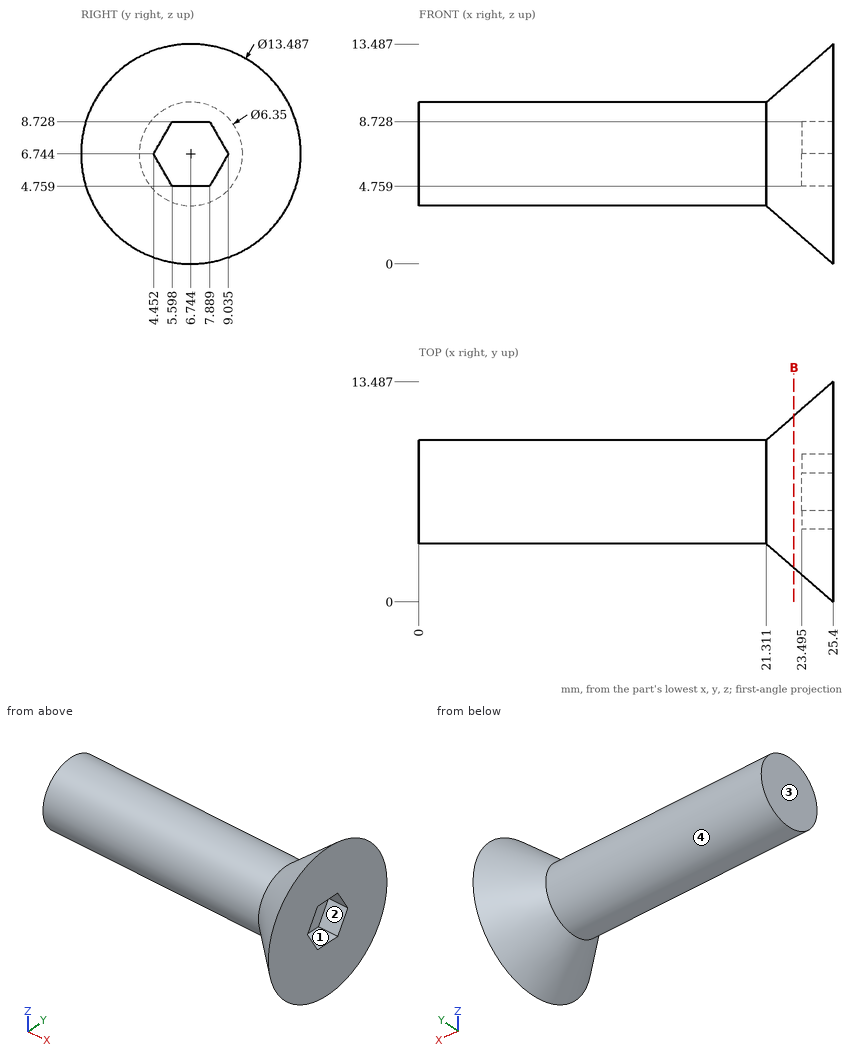
Source: three-view drawing plus pictorial views. Frame: mm from the lowest corner of the part. Give positions to 0.01 mm unless a question says otherwise; leave off trailing zeros. Order: outer loops, then holes, each group sorted by start corner. A loop starts at its lowest first (then second) coordinate and runs counter-clockwise, first axis right, second up. Notation, with made-up numbers: (-37.75, 26.25) - (-13.75, 26.25) arc R26 cw to (-13.75, 49.25) - close; hole circle Ø10 at (-11, 81). An arc over 180 degrees is marked (long way). Answer as a JSON object with one key per item and string values. Group by question number.
Q1. Cut plane B-B, the plane x = 23. Output: boundary loops of the cut face in (y, z), then the cut area to 3 significant figures.
Q2. Mould query, pull axis Z, two halves, no side actions, for the marked faces 1, 2, 3 and 4. Classes: pulls with the +Z half, pulls with the -Z half, needs draft (parallel to the pull), parting line crosses it, or undercut.
Q3. First-contact query: pin 1 Ø3 at (x, z) = (22.5, 8.5) entering from +Y; pin 2 Ø1.5 at (y, z) = (7, 1.5) entering from -X; pin 3 Ø6 at (x, y) = (18, 5.5) entering from +Z. Flat tips, straight axial feed; report the tip coordinate or a pass-through.
Q4. Line query: probe 1 along X at (y, z) = (6.5, 8) (1 decimal); probe 2 along Y at (x, z) = (22, 5) (1 decimal); probe 3 along Y at (x, z) = (7, 6.5). Output: solid intervals per line, ascending.
Results:
{
 "1": {"outline": "circle Ø9.3 at (6.74, 6.74)", "area": "67.9 mm^2"},
 "2": {"face 1": "undercut", "face 2": "undercut", "face 3": "needs draft", "face 4": "parting line crosses it"},
 "3": {"pin 1": "y = 12.05", "pin 2": "x = 22.83", "pin 3": "z = 9.92"},
 "4": {"probe 1": "0 to 23.5", "probe 2": "3.4 to 10.1", "probe 3": "3.58 to 9.91"}
}
